Input: part model. Units: mm. Frame: model coordinates. Face numbers are marked on the shaded views. A direction names the side the tool comes from. Coordinates: 2 decimals unless noted, no trailing zeros. Write each loop counter-clockwise with the first axis right and the second up, starting at its lowest first coordinate (ties: lowest second). Pieces come first, ordered by that corner, then holes. Notation, with made-up numbers: (43.25, -26) - (54.25, -26) arc R11 ccw to (54.25, -13) - close; hole circle Ø8 at (49, -10). An arc over 180 degrees is marked (long way). Use CSV: the item, a comma, the result in double quotes.
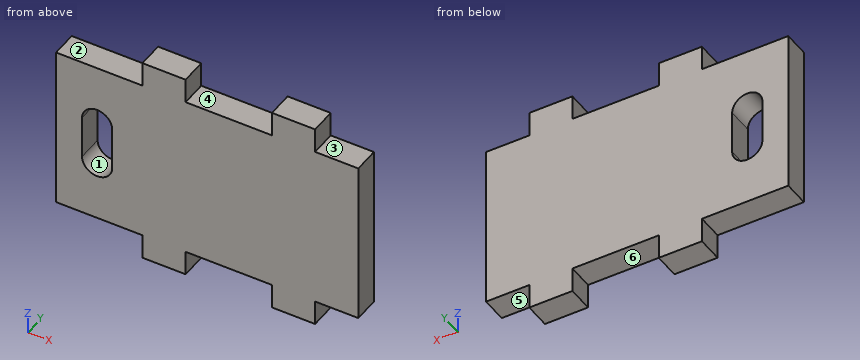
```python
from build123d import *

# Parameters (mm, degrees)
SKETCH1_W           = 60
SKETCH1_H           = 50
BOSS_EXTRUDE1_DEPTH = 6
SKETCH3_W           = 10
SKETCH3_H           = 5.775633532
SKETCH3_W_2         = 20
CUT_EXTRUDE2_DEPTH  = 7
SKETCH4_W           = 10
SKETCH4_H           = 38.448732936
BOSS_EXTRUDE2_DEPTH = 6
CUT_EXTRUDE3_DEPTH  = 7


with BuildPart() as part:
    # Sketch1 → Boss-Extrude1 (new body)
    with BuildSketch(Plane(origin=(0, 0, 0), x_dir=(1, 0, 0), z_dir=(0, 1, 0))):
        with Locations((5, 0)):
            Rectangle(SKETCH1_W, SKETCH1_H)
    extrude(amount=BOSS_EXTRUDE1_DEPTH)

    # Sketch3 → Cut-Extrude2 (cut, through all)
    with BuildSketch(Plane(origin=(0, 6, 0), x_dir=(1, 0, 0), z_dir=(0, 1, 0))):
        with Locations((30, 22.112183234)):
            Rectangle(SKETCH3_W, SKETCH3_H)
        with Locations((5, 22.112183234)):
            Rectangle(SKETCH3_W_2, SKETCH3_H)
        with Locations((-20, 22.112183234)):
            Rectangle(SKETCH3_W, SKETCH3_H)
    cut_extrude2 = extrude(amount=-CUT_EXTRUDE2_DEPTH, mode=Mode.SUBTRACT)

    # Mirror2: Cut-Extrude2 across plane
    add(cut_extrude2.mirror(Plane.XY), mode=Mode.SUBTRACT)

    # Sketch4 → Boss-Extrude2 (add)
    with BuildSketch(Plane(origin=(0, 6, 0), x_dir=(1, 0, 0), z_dir=(0, 1, 0))):
        with Locations((-30, 0)):
            Rectangle(SKETCH4_W, SKETCH4_H)
    extrude(amount=-BOSS_EXTRUDE2_DEPTH)

    # Sketch5 → Cut-Extrude3 (cut, through all)
    with BuildSketch(Plane(origin=(0, 6, 0), x_dir=(1, 0, 0), z_dir=(0, 1, 0))):
        with BuildLine():
            Line((-22, -5), (-22, 5))
            ThreePointArc((-22, 5), (-25.5, 8.5), (-29, 5))
            Line((-29, 5), (-29, -5))
            ThreePointArc((-29, -5), (-25.5, -8.5), (-22, -5))
        make_face()
    extrude(amount=-CUT_EXTRUDE3_DEPTH, mode=Mode.SUBTRACT)


solid = part.part
```
(1) Reachability of the marked faces 1, 2, 3 and 4 from +Z, -Z, +X, -X, +Y, -Y: full face, straight path, thin tool, end or side. Return the list, or none.
Check values:
face 1,"+Y, -Y"
face 2,"+Z, -X, +Y, -Y"
face 3,"+Z, +X, +Y, -Y"
face 4,"+Z, +Y, -Y"
(2) Pin query (flat end, axial travel): pin 1 Ø3 at (x, y) = (1, 4) entering from -Z; pin 2 Ø3 at (x, y) = (30.5, 1.5) entering from +Z; pin 3 Ø1.7 at (y, z) = (4, -22.5) entering from +X. Return the tip coordinate at first contact, or that it passes through.
Check values:
pin 1,"z = -19.22"
pin 2,"z = 19.22"
pin 3,"x = 25"
(3) Cut plane C-C on y = 2.3. Return loops of the section in (x, z).
Check values:
outline,"(-35, -19.22) - (-15, -19.22) - (-15, -25) - (-5, -25) - (-5, -19.22) - (15, -19.22) - (15, -25) - (25, -25) - (25, -19.22) - (35, -19.22) - (35, 19.22) - (25, 19.22) - (25, 25) - (15, 25) - (15, 19.22) - (-5, 19.22) - (-5, 25) - (-15, 25) - (-15, 19.22) - (-35, 19.22) - close; hole (-29, -5) arc R3.5 ccw to (-22, -5) - (-22, 5) arc R3.5 ccw to (-29, 5) - close"
(4) Ray query, probe 1 along X at (y, z) = (1.1, 21); probe 2 along X at (y, z) = (0.6, -4); probe 3 along Z at (x, y) = (3, 0.85). Return the intervals inside material, ascending. Write a range as from..to.
Check values:
probe 1,"-15..-5, 15..25"
probe 2,"-35..-29, -22..35"
probe 3,"-19.22..19.22"
(5) Draft query along X for the marked faces 5 and 6. Return one class per face: pulls with the +X half, pulls with the -X half, needs draft (parallel to the pull), parting line crosses it, or undercut.
Check values:
face 5,"needs draft"
face 6,"undercut"
(6) Cut plane B-B on x = -25.5. Return loops of the section in (y, z).
Check values:
outline,"(0, -19.22) - (6, -19.22) - (6, -8.5) - (0, -8.5) - close; (0, 8.5) - (6, 8.5) - (6, 19.22) - (0, 19.22) - close"
(7) Cut plane D-D on x = 10.5. Return loops of the section in (y, z).
Check values:
outline,"(0, -19.22) - (6, -19.22) - (6, 19.22) - (0, 19.22) - close"
(8) Cut plane A-A on z = 4. Return loops of the section in (x, y).
Check values:
outline,"(-35, 0) - (-29, 0) - (-29, 6) - (-35, 6) - close; (-22, 0) - (35, 0) - (35, 6) - (-22, 6) - close"
